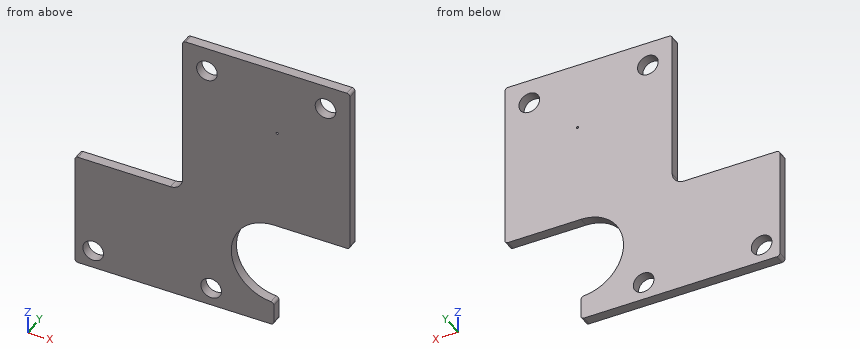
```python
from build123d import *

# Parameters (mm, degrees)
BOSS_EXTRUDE1_DEPTH  = 1.6
FILLET1_R            = 0.5
FILLET2_R            = 2
M3_CLEARANCE_HOLE1_D = 3.4
SKETCH4_R            = 0.175
CUT_EXTRUDE1_DEPTH   = 2.6


with BuildPart() as part:
    # Sketch1 → Boss-Extrude1 (new body)
    with BuildSketch(Plane(origin=(0, 0, 0), x_dir=(1, 0, 0), z_dir=(0, 1, 0))):
        with BuildLine():
            Line((0.032553291, 32.590082792), (0.032553291, 51.590082792))
            Line((0.032553291, 51.590082792), (32.732553291, 51.590082792))
            Line((32.732553291, 51.590082792), (32.732553291, 47.590082792))
            ThreePointArc((32.732553291, 47.590082792), (25.732553291, 40.590082792), (32.732553291, 33.590082792))
            Line((32.732553291, 33.590082792), (45.232553291, 33.590082792))
            Line((45.232553291, 33.590082792), (45.232553291, 5.590082792))
            Line((45.232553291, 5.590082792), (17.732553291, 5.590082792))
            Line((17.732553291, 5.590082792), (17.732553291, 32.590082792))
            Line((17.732553291, 32.590082792), (0.032553291, 32.590082792))
        make_face()
    extrude(amount=BOSS_EXTRUDE1_DEPTH)

    # Fillet1
    fillet1_edges = [part.edges().sort_by_distance(p)[0] for p in [
        (32.732553291, 0.8, -51.590082792),
        (32.732553291, 0.8, -47.590082792),
        (45.232553291, 0.8, -33.590082792),
        (45.232553291, 0.8, -5.590082792),
        (17.732553291, 0.8, -5.590082792),
        (0.032553291, 0.8, -32.590082792),
        (0.032553291, 0.8, -51.590082792),
    ]]
    fillet(fillet1_edges, radius=FILLET1_R)

    # Fillet2
    fillet2_edges = [part.edges().sort_by_distance(p)[0] for p in [
        (17.732553291, 0.8, -32.590082792),
    ]]
    fillet(fillet2_edges, radius=FILLET2_R)

    # M3 Clearance Hole1 (through all)
    with Locations(Plane(origin=(0, 1.6, 0), x_dir=(1, 0, 0), z_dir=(0, 1, 0))):
        with Locations((3.032553291, 48.590082792), (22.432553291, 48.590082792), (21.732553291, 9.590082792), (41.232553291, 9.590082792)):
            Hole(M3_CLEARANCE_HOLE1_D / 2)

    # Sketch4 → Cut-Extrude1 (cut, through all)
    with BuildSketch(Plane(origin=(0, 1.6, 0), x_dir=(1, 0, 0), z_dir=(0, 1, 0))):
        with Locations((33.297557825, 16.825078258)):
            Circle(SKETCH4_R)
    extrude(amount=-CUT_EXTRUDE1_DEPTH, mode=Mode.SUBTRACT)


solid = part.part
```
Model file for the job. Use its own axes, mm. Coordinates: 2 decimals unless noted, no trailing zeros. Order: outer loops, then holes, each group sorted by start corner. A loop starts at its lowest first (then second) coordinate and runs counter-clockwise, first axis right, second up. Notation, with made-up numbers: (32, 50) -> (42, 50) arc R13 cw to (42, 56) -> close; hole circle Ø3 at (10, 7.5). An arc over 180 degrees is marked (long way). Return JSON: item names as keys, results as strings.
Item 1: Slice it at D-D (x = 28). Write the cut outline in (y, z), then the cut area to 3 significant figures.
Model answer:
{"outline": "(0, -51.59) -> (1.6, -51.59) -> (1.6, -45.75) -> (0, -45.75) -> close; (0, -35.43) -> (1.6, -35.43) -> (1.6, -5.59) -> (0, -5.59) -> close", "area": "57.1 mm²"}
Item 2: Slice it at B-B (z = -29). Write the cut outline in (x, y), then the cut area to 3 significant figures.
Model answer:
{"outline": "(17.73, 0) -> (45.23, 0) -> (45.23, 1.6) -> (17.73, 1.6) -> close", "area": "44.0 mm²"}
Item 3: Wall check: line 1 along X through (y, z) = (0.7, -9); line 2 along Z through (x, y) = (7, 1.15); line 3 along X through (y, z) = (1, -20). Give the ranges that are in metal, low to high. Write a range as from..to.
Model answer:
{"line 1": "x = 17.73..20.14, 23.33..39.64, 42.83..45.23", "line 2": "z = -51.59..-32.59", "line 3": "x = 17.73..45.23"}
Item 4: Slice it at A-A (x = 4). Write the cut outline in (y, z), then the cut area to 3 significant figures.
Model answer:
{"outline": "(0, -51.59) -> (1.6, -51.59) -> (1.6, -49.99) -> (0, -49.99) -> close; (0, -47.19) -> (1.6, -47.19) -> (1.6, -32.59) -> (0, -32.59) -> close", "area": "25.9 mm²"}
Item 5: Slice it at C-C (y = 1.15). Count the separate pieces of the cut face and the enclosed holes in it, then the cut area to 3 significant figures.
Model answer:
{"separate pieces": "1", "enclosed holes": "5", "area": "1,260 mm²"}
Item 6: Pin check, flat tips, straight feed: P1, Ø0.8, axis at y = 0.5, z = -18, coming from the -X side; P2, Ø3, axis at x = 41.23, z = -9.59, coming from the -Y side; P3, Ø0.5, axis at x = 38, y = 1, coming from the -Z side. Stop position of each tip, or through.
Model answer:
{"P1": "stops at x = 17.73", "P2": "passes through", "P3": "stops at z = -33.59"}
